Can you work these out from the model? Positions are in its coordinate system, mm. A direction names the side the tool comes from. Round coordinates to 2 decimals unless told otherwise and drop trailing zeros. Write each loop counter-clockwise with the first axis right and the second up, starting at its lowest first coordinate (ties: lowest second). Pieces come first, ordered by that corner, then holes. Notation, with made-up numbers: (73.25, 55) -> (97.25, 55) arc R20 cw to (97.25, 67) -> close; hole circle Ø5 at (2, 24). An arc over 180 degrees is marked (long way). Write item = value, one per line. Start each with the question number.
1) I'm going to push flat-ended pins straight in: pin 1 (15 mm diameter, centred on y = -8.5, z = -6.5, fed in from -X); pin 2 (9.5 mm diameter, centred on y = -11.5, z = 13, fed in from +X). Where does each tip first touch, or does it pass through?
2) If I drill on line 1 (X direction, y = -1.5, z = 5), over which ranges is the centre line in solid material (lowest first)?
3) Imagine slicing it at A-A, the plane z = -22. Please give me the cut outline in (x, y).
4) Imagine slicing it at B-B, the plane y = -9.5. Please give me the cut outline in (x, z).
5) For faces 1 (the face through (895, 0, 1)), 2 (the face through (13, 19.05, -1)), 3 (the face through (-895, 0, 1)), which set-ups out of +Z, -Z, +X, -X, +Y, -Y let a thin tool reach every point of the face, with its end or its side?
from build123d import *

# Parameters (mm, degrees)
F0_W     = 38.1
F0_H     = 88.9
F1_DEPTH = 939.8
F2_W     = 88.9
F2_H     = 19.05
F3_DEPTH = 88.9


with BuildPart() as f1:
    # F0 (on Right) → F1 (new body)
    with BuildSketch(Plane.YZ):
        Rectangle(F0_W, F0_H)
    extrude(amount=F1_DEPTH)

    # F2 (on face) → F3 (cut, through all)
    with BuildSketch(Plane.XY.offset(44.45)):
        with Locations((895.35, -9.525)):
            Rectangle(F2_W, F2_H)
    extrude(amount=-F3_DEPTH, mode=Mode.SUBTRACT)

    # F4: F1 across plane


with BuildPart() as f1_1:
    add(f1.part)
    add(f1.part.mirror(Plane.YZ))


solid = f1_1.part
Reported:
q1.pin_1 = -850.9
q1.pin_2 = 850.9
q2.line_1 = -850.9 to 850.9
q3.outline = (-939.8, 0) -> (-850.9, 0) -> (-850.9, -19.05) -> (850.9, -19.05) -> (850.9, 0) -> (939.8, 0) -> (939.8, 19.05) -> (-939.8, 19.05) -> close
q4.outline = (-850.9, -44.45) -> (850.9, -44.45) -> (850.9, 44.45) -> (-850.9, 44.45) -> close
q5.face_1 = +Z, -Z, +X, -Y
q5.face_2 = +Z, -Z, +X, -X, +Y
q5.face_3 = +Z, -Z, -X, -Y
